Work out the finished part from the listing and answer in its coordinate system (mm). Face numbers are marked on the shaded views. A direction names the side the tool comes from. Give positions to 0.01 mm unless a question says otherwise; leave off trailing zeros. Loops run counter-clockwise (first coordinate to the right, second up) from the corner with the lowest first, then second, coordinate; pieces in that order, holes last. Notation, with made-up numbers: (59.5, -22) - (102.5, -22) arc R11 cw to (102.5, -13) - close; hole circle Ø10 at (-21, 89.5). An arc over 180 degrees is marked (long way). One line per item, written item: value.
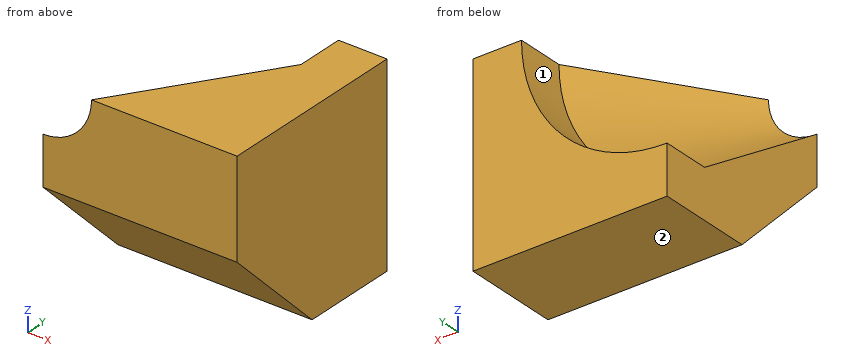
from build123d import *

# Parameters (mm, degrees)
SKETCH1_W           = 40
SKETCH1_H           = 40
BOSS_EXTRUDE1_DEPTH = 40
CUT_EXTRUDE1_DEPTH  = 40
CUT_EXTRUDE2_DEPTH  = 40
CUT_EXTRUDE3_DEPTH  = 10
BOSS_EXTRUDE2_DEPTH = 28
CUT_EXTRUDE11_DEPTH = 10
SKETCH20_W          = 40
SKETCH20_H          = 20
CUT_EXTRUDE12_DEPTH = 10
SKETCH21_W          = 40
SKETCH21_H          = 28.284271248
CUT_EXTRUDE13_DEPTH = 10
CUT_EXTRUDE14_DEPTH = 10
SKETCH23_W          = 40
SKETCH23_H          = 40
CUT_EXTRUDE15_DEPTH = 10
SKETCH24_W          = 40
SKETCH24_H          = 40
CUT_EXTRUDE16_DEPTH = 10
CUT_EXTRUDE17_DEPTH = 59
CUT_EXTRUDE18_DEPTH = 59


with BuildPart() as part:
    # Sketch1 → Boss-Extrude1 (new body)
    with BuildSketch(Plane.XY):
        with Locations((20, 20)):
            Rectangle(SKETCH1_W, SKETCH1_H)
    extrude(amount=BOSS_EXTRUDE1_DEPTH)

    # Sketch2 → Cut-Extrude1 (cut)
    with BuildSketch(Plane(origin=(0, 40, 0), x_dir=(1, 0, 0), z_dir=(0, 1, 0))):
        with BuildLine():
            Line((0, -30), (0, -40))
            Line((0, -40), (10, -40))
            ThreePointArc((10, -40), (7.071067812, -32.928932188), (0, -30))
        make_face()
    extrude(amount=-CUT_EXTRUDE1_DEPTH, mode=Mode.SUBTRACT)

    # Sketch3 → Cut-Extrude2 (cut)
    with BuildSketch(Plane(origin=(40, 0, 0), x_dir=(0, 0, -1), z_dir=(1, 0, 0))):
        Polygon((0, 20), (-20, 0), (0, 0), align=None)
    extrude(amount=-CUT_EXTRUDE2_DEPTH, mode=Mode.SUBTRACT)

    # Sketch4 → Cut-Extrude3 (cut)
    with BuildSketch(Plane(origin=(0, 40, 0), x_dir=(1, 0, 0), z_dir=(0, 1, 0))):
        with BuildLine():
            Line((0, -10), (0, -30))
            ThreePointArc((0, -30), (7.071067812, -32.928932188), (10, -40))
            Line((10, -40), (30, -40))
            ThreePointArc((30, -40), (21.213203436, -18.786796564), (0, -10))
        make_face()
    extrude(amount=-CUT_EXTRUDE3_DEPTH, mode=Mode.SUBTRACT)

    # Sketch8 → Boss-Extrude2 (add)
    with BuildSketch(Plane(origin=(-13.333333333, 6.666666667, 13.333333333), x_dir=(-0.745355992, -0.298142397, -0.596284794), z_dir=(0.666666667, -0.333333333, -0.666666667))):
        Polygon((-17.88854382, 31.304951685), (-17.88854382, -13.416407865), (-31.304951685, -17.88854382), (-58.137767415, 17.88854382), align=None)
    extrude(amount=BOSS_EXTRUDE2_DEPTH)

    # Sketch19 → Cut-Extrude11 (cut)
    with BuildSketch(Plane(origin=(0, 40, 0), x_dir=(1, 0, 0), z_dir=(0, 1, 0))):
        with BuildLine():
            Line((0, -10), (0, -40))
            Line((0, -40), (30, -40))
            ThreePointArc((30, -40), (21.213203436, -18.786796564), (0, -10))
        make_face()
    extrude(amount=-CUT_EXTRUDE11_DEPTH, mode=Mode.SUBTRACT)

    # Sketch20 → Cut-Extrude12 (cut)
    with BuildSketch(Plane(origin=(0, 0, 0), x_dir=(-1, 0, 0), z_dir=(0, 0, -1))):
        with Locations((-20, 30)):
            Rectangle(SKETCH20_W, SKETCH20_H)
    extrude(amount=CUT_EXTRUDE12_DEPTH, mode=Mode.SUBTRACT)

    # Sketch21 → Cut-Extrude13 (cut)
    with BuildSketch(Plane(origin=(0, 10, 10), x_dir=(1, 0, 0), z_dir=(0, -0.707106781, -0.707106781))):
        with Locations((20, 0)):
            Rectangle(SKETCH21_W, SKETCH21_H)
    extrude(amount=CUT_EXTRUDE13_DEPTH, mode=Mode.SUBTRACT)

    # Sketch22 → Cut-Extrude14 (cut)
    with BuildSketch(Plane(origin=(0, 10, -10), x_dir=(1, 0, 0), z_dir=(0, -0.707106781, 0.707106781))):
        Polygon((16, 14.142135624), (22, 14.142135624), (18.666666667, 10.999438818), align=None)
    extrude(amount=-CUT_EXTRUDE14_DEPTH, mode=Mode.SUBTRACT)

    # Sketch23 → Cut-Extrude15 (cut)
    with BuildSketch(Plane.XZ):
        with Locations((20, 20)):
            Rectangle(SKETCH23_W, SKETCH23_H)
    extrude(amount=CUT_EXTRUDE15_DEPTH, mode=Mode.SUBTRACT)

    # Sketch24 → Cut-Extrude16 (cut)
    with BuildSketch(Plane(origin=(40, 0, 0), x_dir=(0, 0, -1), z_dir=(1, 0, 0))):
        with Locations((-20, 20)):
            Rectangle(SKETCH24_W, SKETCH24_H)
    extrude(amount=CUT_EXTRUDE16_DEPTH, mode=Mode.SUBTRACT)

    # Sketch25 → Cut-Extrude17 (cut)
    with BuildSketch(Plane(origin=(-12.272727273, 8.181818182, 12.272727273), x_dir=(0.768706115, 0.354787438, 0.532181156), z_dir=(-0.639602149, 0.426401433, 0.639602149))):
        Polygon((15.965434692, -16.641005887), (15.965434692, 19.414506868), (54.992052827, 2.773500981), (28.974307403, -22.188007849), align=None)
    extrude(amount=CUT_EXTRUDE17_DEPTH, mode=Mode.SUBTRACT)

    # Sketch26 → Cut-Extrude18 (cut)
    with BuildSketch(Plane(origin=(0, 30, 0), x_dir=(1, 0, 0), z_dir=(0, 1, 0))):
        with BuildLine():
            Line((0, -30), (0, -40))
            Line((0, -40), (10, -40))
            ThreePointArc((10, -40), (7.071067812, -32.928932188), (0, -30))
        make_face()
    extrude(amount=-CUT_EXTRUDE18_DEPTH, mode=Mode.SUBTRACT)

    # Sketch27 → Cut-Revolve1 (revolve, cut)
    with BuildSketch(Plane.XY.offset(40)):
        Polygon((30, 30), (10, 0), (10, 30), align=None)
    revolve(axis=Axis((0, 0, 40), (0, 1, 0)), mode=Mode.SUBTRACT)


solid = part.part
1. Section A-A (y = 31) is taken. Write down the section's boundary in (x, z), and give its area (3 significant figures).
Output:
outline: (0, 0) - (40, 0) - (40, 40) - (30, 40) arc R30 cw to (0, 10) - close
area: 893 mm²
2. Section B-B (z = 6) is taken. Write down the section's boundary in (x, y), and give its area (3 significant figures).
Output:
outline: (0, 14) - (40, 14) - (40, 40) - (0, 40) - close
area: 1,040 mm²
3. For the marked faces 1 and 2, determine the directions among +Z, -Z, +X, -X, +Y, -Y from which every point of the face is accessible in a straight line to the end or side of a thin tool.
Output:
face 1: +Z, -X, +Y
face 2: -Z, +X, -X, +Y, -Y
4. Section C-C (x = 35) is taken. Write down the section's boundary in (y, z), and give its area (3 significant figures).
Output:
outline: (0, 20) - (20, 0) - (40, 0) - (40, 40) - (0, 40) - close
area: 1,400 mm²
5. Flat-ended cylindrical pins translate along their axes: pin 1 Ø1 at (x, y) = (22, 23.5) entering from +Z; pin 2 Ø2 at (x, y) = (32.5, 4.5) entering from -Z; pin 3 Ø1 at (y, z) = (16, 33.5) entering from -X. Find the tip coordinate at first contact, or state that the pin passes through.
Output:
pin 1: stops at z = 27.88
pin 2: stops at z = 14.5
pin 3: stops at x = 19.23
6. Find the intervals of material crossed by line 1 along Y through (x, z) = (2, 14.5); line 2 along X through (y, z) = (29, 21); line 3 along Z through (x, y) = (21, 38), in increasing order.
Output:
line 1: y = 5.5 to 23.37
line 2: x = 22.35 to 40
line 3: z = 0 to 18.58
